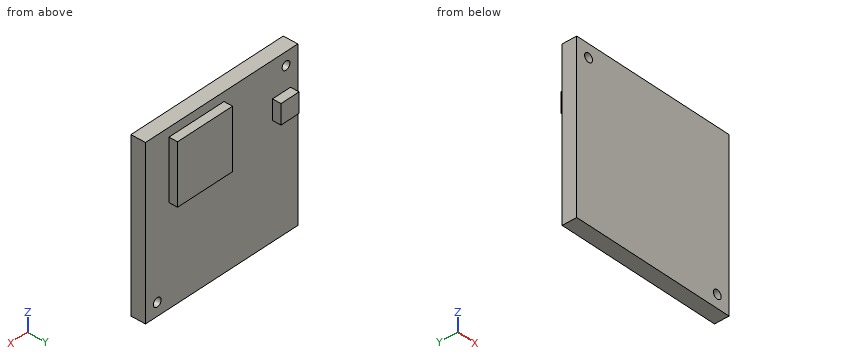
```python
from build123d import *

# Parameters (mm, degrees)
SKETCH1_W           = 19.4
SKETCH1_H           = 19.4
SKETCH1_R           = 0.5
BOSS_EXTRUDE1_DEPTH = 1.7
SKETCH2_W           = 7
SKETCH2_H           = 7
SKETCH2_W_2         = 2.3
SKETCH2_H_2         = 2.3
BOSS_EXTRUDE2_DEPTH = 1


with BuildPart() as part:
    # Sketch1 → Boss-Extrude1 (new body)
    with BuildSketch(Plane(origin=(0, 0, 0), x_dir=(1, 0, 0), z_dir=(0, 1, 0))):
        Rectangle(SKETCH1_W, SKETCH1_H)
        with Locations(Location((-8.2, -8.2, 0), (0, 0, 270))):
            Circle(SKETCH1_R, mode=Mode.SUBTRACT)
        with Locations(Location((8.2, 8.2, 0), (0, 0, 270))):
            Circle(SKETCH1_R, mode=Mode.SUBTRACT)
    extrude(amount=BOSS_EXTRUDE1_DEPTH)

    # Sketch2 → Boss-Extrude2 (add)
    with BuildSketch(Plane(origin=(0, 1.7, 0), x_dir=(1, 0, 0), z_dir=(0, 1, 0))):
        with Locations((3.206065648, -5.151943642)):
            Rectangle(SKETCH2_W, SKETCH2_H)
        with Locations((-7.616722435, -4.429188959)):
            Rectangle(SKETCH2_W_2, SKETCH2_H_2)
    extrude(amount=BOSS_EXTRUDE2_DEPTH)


solid = part.part
```
The model under review builds one solid part; all positions refer to its coordinate system, in mm. Coordinates: 2 decimals unless noted, no trailing zeros. Write each loop counter-clockwise with the first axis right and the second up, starting at its lowest first coordinate (ties: lowest second). Pieces come first, ordered by that corner, then holes. Notation, with made-up numbers: (-12, -35) - (44, -35) arc R19 cw to (44, -11) - close; hole circle Ø5 at (51, -9). An arc over 180 degrees is marked (long way). Write item = value, one per line.
(1) Consider section B-B, the plane z = -8.2. Give the boundary of the cut face in (x, y).
Result sheet:
outline = (-9.7, 0) - (7.7, 0) - (7.7, 1.7) - (-9.7, 1.7) - close; (8.7, 0) - (9.7, 0) - (9.7, 1.7) - (8.7, 1.7) - close
(2) Consider section C-C, the plane x = -8.2. Give the boundary of the cut face in (y, z), then the cut area to 3 significant figures.
Result sheet:
outline = (0, -9.7) - (1.7, -9.7) - (1.7, 3.28) - (2.7, 3.28) - (2.7, 5.58) - (1.7, 5.58) - (1.7, 7.7) - (0, 7.7) - close; (0, 8.7) - (1.7, 8.7) - (1.7, 9.7) - (0, 9.7) - close
area = 33.6 mm^2
(3) For line 1 (X direction, y = 0.4, z = -8.2); line 2 (Y direction, x = -6.75, z = -8); line 3 (X direction, y = 0.5, z = 8.2), list the stretches that pass through material, from the lowest coordinate up. Write a range as [from, to].
Result sheet:
line_1 = [-9.7, 7.7], [8.7, 9.7]
line_2 = [0, 1.7]
line_3 = [-9.7, -8.7], [-7.7, 9.7]
(4) Consider section A-A, the plane y = 1.95. Give the boundary of the cut face in (x, z).
Result sheet:
outline = (-8.77, 3.28) - (-6.47, 3.28) - (-6.47, 5.58) - (-8.77, 5.58) - close; (-0.29, 1.65) - (6.71, 1.65) - (6.71, 8.65) - (-0.29, 8.65) - close
(5) Consider section D-D, the plane z = 4. Give the boundary of the cut face in (x, y).
Result sheet:
outline = (-9.7, 0) - (9.7, 0) - (9.7, 1.7) - (6.71, 1.7) - (6.71, 2.7) - (-0.29, 2.7) - (-0.29, 1.7) - (-6.47, 1.7) - (-6.47, 2.7) - (-8.77, 2.7) - (-8.77, 1.7) - (-9.7, 1.7) - close
(6) For P1, Ø2, axis at x = -3.5, z = -7, coming from the +Y side; P2, Ø0.8, axis at x = 2, y = 2.5, coming from the +Z side; P3, Ø0.5, axis at x = -7.5, y = 2, coming from the -Z side, all flat-tipped, find the tip position at first contact; note any pin that passes through.
Result sheet:
P1 = 1.7
P2 = 8.65
P3 = 3.28
